from build123d import *

# Parameters (mm, degrees)
SKETCH1_R               = 11
BOSS_EXTRUDE1_DEPTH     = 30.4
CUT_EXTRUDE1_DEPTH      = 65.4
CUT_EXTRUDE1_DEPTH_BACK = 30.4
SKETCH2_R               = 2.5
SKETCH2_W               = 60.96
SKETCH2_H               = 5
SKETCH3_R               = 1.016
BOSS_EXTRUDE2_DEPTH     = 2.54


with BuildPart() as part:
    # Sketch1 → Boss-Extrude1 (new body)
    with BuildSketch(Plane.XY):
        with BuildLine():
            Line((-40.64, -29.21), (40.64, -29.21))
            Line((40.64, -29.21), (40.64, -25.4))
            Line((40.64, -25.4), (15.24, -25.4))
            Line((15.24, -25.4), (15.24, 0))
            ThreePointArc((15.24, 0), (0, 15.24), (-15.24, 0))
            Line((-15.24, 0), (-15.24, -25.4))
            Line((-15.24, -25.4), (-40.64, -25.4))
            Line((-40.64, -25.4), (-40.64, -29.21))
        make_face()
        with Locations(Location((0, 0, 0), (0, 0, 180))):
            Circle(SKETCH1_R, mode=Mode.SUBTRACT)
    extrude(amount=BOSS_EXTRUDE1_DEPTH)

    # Sketch2 → Cut-Extrude1 (cut, two sides: drawn at the far end of the back side and taken through both)
    with BuildSketch(Plane(origin=(0, -25.4, 0), x_dir=(1, 0, 0), z_dir=(0, 1, 0)).offset(-CUT_EXTRUDE1_DEPTH_BACK)):
        with Locations(Location((-36.14, -5, 0), (0, 0, 90))):
            Circle(SKETCH2_R)
        with Locations(Location((-35, -18.4, 0), (0, 0, 90))):
            Circle(SKETCH2_R)
        with Locations(Location((36.14, -5, 0), (0, 0, 90))):
            Circle(SKETCH2_R)
        with Locations(Location((35, -18.4, 0), (0, 0, 90))):
            Circle(SKETCH2_R)
        with Locations((0, -2.5)):
            Rectangle(SKETCH2_W, SKETCH2_H)
    extrude(amount=CUT_EXTRUDE1_DEPTH + CUT_EXTRUDE1_DEPTH_BACK, mode=Mode.SUBTRACT)

    # Sketch3 → Boss-Extrude2 (add)
    with BuildSketch(Plane(origin=(0, 0, 5), x_dir=(-1, 0, 0), z_dir=(0, 0, -1))):
        with BuildLine():
            Line((0, 11), (0, 15.24))
            Line((0, 15.24), (30.48, 15.24))
            Line((30.48, 15.24), (30.48, -25.4))
            Line((30.48, -25.4), (0, -25.4))
            Line((0, -25.4), (0, -11))
            ThreePointArc((0, -11), (11, 0), (0, 11))
        make_face()
        with Locations((28.1178, 10.4775)):
            Circle(SKETCH3_R, mode=Mode.SUBTRACT)
        with Locations((28.1178, -10.4775)):
            Circle(SKETCH3_R, mode=Mode.SUBTRACT)
    extrude(amount=-BOSS_EXTRUDE2_DEPTH)


solid = part.part
Geometry: final body of the model. Coordinates: model frame, mm. A direction names the side the tool comes from. Coordinates: 2 decimals unless noted, no trailing zeros. Write each loop counter-clockwise with the first axis right and the second up, starting at its lowest first coordinate (ties: lowest second). Pieces come first, ordered by that corner, then holes. Notation, with made-up numbers: (69, 72) - (93, 72) arc R17 ccw to (93, 98) - close; hole circle Ø5 at (45.5, 3). An arc over 180 degrees is marked (long way). Return JSON: item names as keys, results as strings.
Item 1: Pin query (flat end, axial travel): pin 1 Ø6 at (x, z) = (-35, 18.4) entering from +Y; pin 2 Ø12 at (x, y) = (-5.5, -13.5) entering from -Z; pin 3 Ø4 at (y, z) = (-16.5, 16.5) entering from +X. Return the tip coordinate at first contact, or that it passes through.
Completed:
{"pin 1": "stops at y = -25.4", "pin 2": "stops at z = 5", "pin 3": "stops at x = 15.24"}
Item 2: Reachability of faces 4 (the face through (30.48, -27, 3)), 5 (the face through (28, -25.4, 18)), 6 (the face through (-15.24, -13, 19)) from +Z, -Z, +X, -X, +Y, -Y: full face, straight path, thin tool, end or side. Return the list, or none.
Completed:
{"face 4": "-Z, +Y, -Y", "face 5": "+Z, -Z, +X, +Y", "face 6": "+Z, -X, +Y"}
Item 3: Section query B-B (y = -6.5). Output: boundary loops of the cut face in (x, z).
Completed:
{"outline": "(-30.48, 5) - (-8.87, 5) - (-8.87, 30.4) - (-15.24, 30.4) - (-15.24, 7.54) - (-30.48, 7.54) - close; (8.87, 5) - (15.24, 5) - (15.24, 30.4) - (8.87, 30.4) - close"}
Item 4: Section query C-C (z = 6). Output: boundary loops of the cut face in (x, y), and give its area (3 significant figures).
Completed:
{"outline": "(-40.64, -29.21) - (-38.43, -29.21) - (-38.43, -25.4) - (-40.64, -25.4) - close; (-33.85, -29.21) - (33.85, -29.21) - (33.85, -25.4) - (15.24, -25.4) - (15.24, 0) arc R15.24 ccw to (0, 15.24) - (-30.48, 15.24) - (-30.48, -25.4) - (-33.85, -25.4) - close; (38.43, -29.21) - (40.64, -29.21) - (40.64, -25.4) - (38.43, -25.4) - close; hole circle Ø2.03 at (-28.12, -10.48); hole circle Ø2.03 at (-28.12, 10.48); hole circle Ø22 at (0, 0)", "area": "1,700 mm2"}
Item 5: Line query: L1, parallel to X at y = 0.5, z = 23.5; L2, parallel to Y at x = -35.5, z = 2.5; L3, parallel to Z at x = -28.5, y = 8.5. Output: solid intervals per line, ascending.
Completed:
{"L1": "x = -15.23 to -10.99, 10.99 to 15.23", "L2": "y = -29.21 to -25.4", "L3": "z = 5 to 7.54"}
Item 6: Section query A-A (z = 18.4). Output: boundary loops of the cut face in (x, y), and give its area (3 significant figures).
Completed:
{"outline": "(-40.64, -29.21) - (-37.5, -29.21) - (-37.5, -25.4) - (-40.64, -25.4) - close; (-32.5, -29.21) - (32.5, -29.21) - (32.5, -25.4) - (15.24, -25.4) - (15.24, 0) arc R15.24 ccw to (-15.24, 0) - (-15.24, -25.4) - (-32.5, -25.4) - close; (37.5, -29.21) - (40.64, -29.21) - (40.64, -25.4) - (37.5, -25.4) - close; hole circle Ø22 at (0, 0)", "area": "1,030 mm2"}
Item 7: Pull-direction query (Z, two-part tool) for faces 1 (the face through (-40.64, -27, 15)), 2 (the face through (35, -27, 0)), 3 (the face through (33.31, -27.33, 20.24)); classes: +Z half, -Z half, draft (parallel to the pull), parting line (faces both ways), or undercut.
Completed:
{"face 1": "draft", "face 2": "-Z half", "face 3": "undercut"}
Item 8: Section query D-D (x = -36.14). Output: boundary loops of the cut face in (y, z), and give its area (3 significant figures).
Completed:
{"outline": "(-29.21, 0) - (-25.4, 0) - (-25.4, 2.5) - (-29.21, 2.5) - close; (-29.21, 7.5) - (-25.4, 7.5) - (-25.4, 16.18) - (-29.21, 16.18) - close; (-29.21, 20.62) - (-25.4, 20.62) - (-25.4, 30.4) - (-29.21, 30.4) - close", "area": "79.8 mm2"}
